Geometry check sheet. Reference: drawing and pictorial views, mm from the part's lowest x, y, z. A direction names the side the tool comes from. Coordinates: 2 decimals unless noted, no trailing zeros. Write each loop counter-clockwise with the first axis right and the second up, starting at its lowest first coordinate (ties: lowest second). Pieces come first, ordered by that corner, then holes.
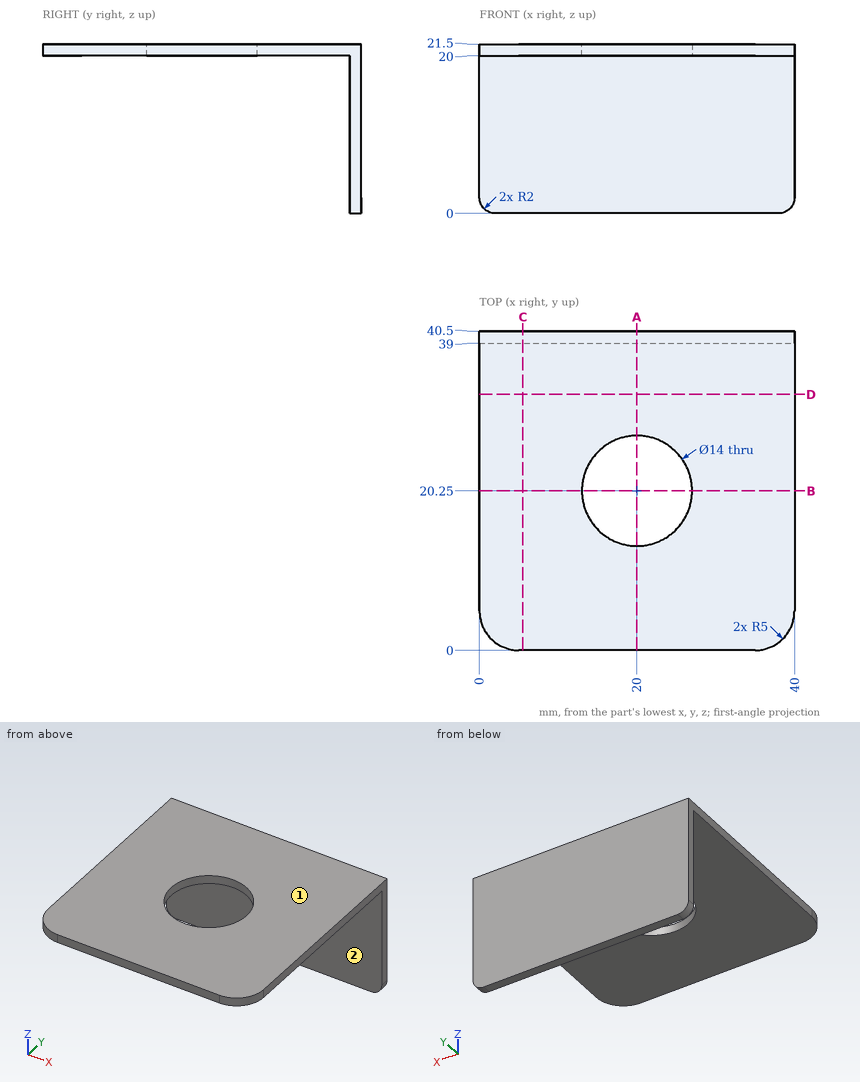
1. Gauge pin test, flat ends, axial feed: P1, Ø6, axis at x = 17.5, z = 10.5, coming from the -Y side; P2, Ø11.5, axis at x = 13.5, y = 22, coming from the -Z side. Record the tip position at first contact, or that the pin passes through.
2. Sectioned sample at B-B, the plane y = 20.25. Record the boundary of the cut face in (x, z), and give its area (3 significant figures).
3. Material ranges on L1, parallel to Y at x = 20, z = 20.75; L2, parallel to Z at x = 28, y = 26; L3, parallel to Y at x = 11, z = 19, recorded low to high.
4. Sectioned sample at A-A, the plane x = 20. Record the boundary of the cut face in (y, z).
5. Tool access check on the marked faces 1 and 2. Record the directions out of +Z, -Z, +X, -X, +Y, -Y that give a thin tool (end or side, any length) a straight path to the whole face; none if there is none.
6. Sectioned sample at D-D, the plane y = 32.5. Record the boundary of the cut face in (x, z), and give its area (3 significant figures).
7. Sectioned sample at C-C, the plane x = 5.5. Record the boundary of the cut face in (y, z), and give its area (4 significant figures).
Outcome:
1. P1: stops at y = 39
1. P2: stops at z = 20
2. outline: (0, 20) - (13, 20) - (13, 21.5) - (0, 21.5) - close; (27, 20) - (40, 20) - (40, 21.5) - (27, 21.5) - close
2. area: 39.0 mm2
3. L1: y = 0 to 13.25, 27.25 to 40.5
3. L2: z = 20 to 21.5
3. L3: y = 39 to 40.5
4. outline: (0, 20) - (13.25, 20) - (13.25, 21.5) - (0, 21.5) - close; (27.25, 20) - (39, 20) - (39, 0) - (40.5, 0) - (40.5, 21.5) - (27.25, 21.5) - close
5. face 1: +Z, +X, -X, +Y, -Y
5. face 2: -Z, +X, -X, -Y
6. outline: (0, 20) - (40, 20) - (40, 21.5) - (0, 21.5) - close
6. area: 60.0 mm2
7. outline: (0, 20) - (39, 20) - (39, 0) - (40.5, 0) - (40.5, 21.5) - (0, 21.5) - close
7. area: 90.75 mm2
